```python
from build123d import *

# Parameters (mm, degrees)
F0_R     = 4
F1_DEPTH = 40


with BuildPart() as f1:
    # F0 (on Front) → F1 (new body)
    with BuildSketch(Plane.XZ):
        with BuildLine():
            ThreePointArc((-5.386362, 16.181819), (-8.921896, 17.646285), (-10.386362, 21.181819))
            Line((-10.386362, 21.181819), (-10.386362, 16.181819))
            Line((-10.386362, 16.181819), (-5.386362, 16.181819))
        make_face()
        with BuildLine():
            ThreePointArc((-5.386362, 16.181819), (-1.850828, 17.646285), (-0.386362, 21.181819))
            ThreePointArc((-0.386362, 21.181819), (-5.386362, 26.181819), (-10.386362, 21.181819))
            ThreePointArc((-10.386362, 21.181819), (-8.921896, 17.646285), (-5.386362, 16.181819))
        make_face()
        with Locations((-5.386362, 21.181819)):
            Circle(F0_R, mode=Mode.SUBTRACT)
        with BuildLine():
            Line((-0.386362, 16.181819), (-0.386362, 21.181819))
            ThreePointArc((-0.386362, 21.181819), (-1.850828, 17.646285), (-5.386362, 16.181819))
            Line((-5.386362, 16.181819), (-0.386362, 16.181819))
        make_face()
    extrude(amount=F1_DEPTH)


solid = f1.part
```
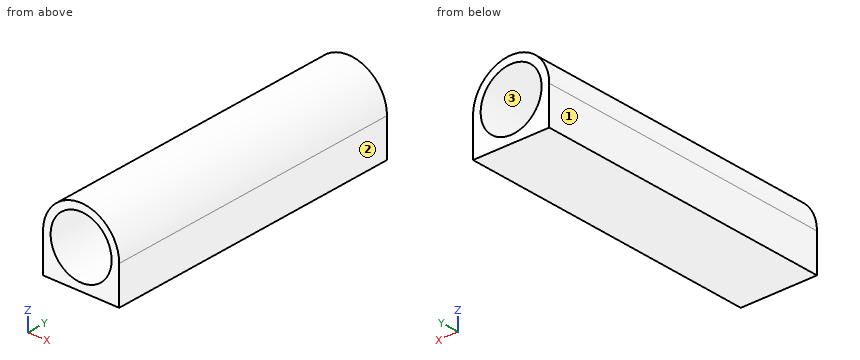
Geometry check sheet. Reference: the model listing, model coordinates, mm. Face numbers are marked on the shaded views. Coordinates: 2 decimals unless noted, no trailing zeros. Write each loop counter-clockwise with the first axis right and the second up, starting at its lowest first coordinate (ties: lowest second). Pieces come first, ordered by that corner, then holes. Notation, with made-up numbers: M 78,74.25 L 121,74.25 A14 ccw 121,79.25 Z; hole C -2,13 d4. An arc over 180 degrees is marked long. Use one line per item in the form item = value. Start each with the question number.
1) Section check C-C on y = -31. Enter the section's corners in (x, z), and give its area (3 significant figures).
2) Go/stop test with a flat-tipped pin: pin 1 Ø2 at (x, z) = (-6.5, 20) entering from -Y. Record where the tip stops, or that it passes through.
3) Thickness scan on probe 1 along Z at (x, y) = (-5.25, -20); probe 2 along X at (y, z) = (-4, 21); probe 3 along X at (y, z) = (-37, 22.5). Record the ranges inside material, lowest first. Write a range as from..to.
4) Section check B-B on x = -4.75. Enter the section's corners in (y, z).
5) Section check D-D on z = 25.75. Enter the section's corners in (x, y).
6) Release check for a two-part mould opening along X. For the marked faces 1, 2 and 3 record: pulls with the +X half, pulls with the -X half, needs draft (parallel to the pull), parting line crosses it, or undercut.
7) Section check A-A on z = 24.25. Enter the section's corners in (x, y), and give its area (3 significant figures).
Responses:
q1.outline = M -10.39,16.18 L -0.39,16.18 L -0.39,21.18 A5 ccw -10.39,21.18 Z; hole C -5.39,21.18 d8
q1.area = 39.0 mm2
q2.pin_1 = through
q3.probe_1 = 16.18..17.18, 25.18..26.18
q3.probe_2 = -10.39..-9.38, -1.39..-0.39
q3.probe_3 = -10.21..-9.16, -1.61..-0.56
q4.outline = M -40,16.18 L 0,16.18 L 0,17.23 L -40,17.23 Z; M -40,25.13 L 0,25.13 L 0,26.14 L -40,26.14 Z
q5.outline = M -7.42,-40 L -3.35,-40 L -3.35,0 L -7.42,0 Z
q6.face_1 = pulls with the -X half
q6.face_2 = pulls with the +X half
q6.face_3 = undercut
q7.outline = M -9.33,-40 L -7.95,-40 L -7.95,0 L -9.33,0 Z; M -2.82,-40 L -1.44,-40 L -1.44,0 L -2.82,0 Z
q7.area = 111 mm2
